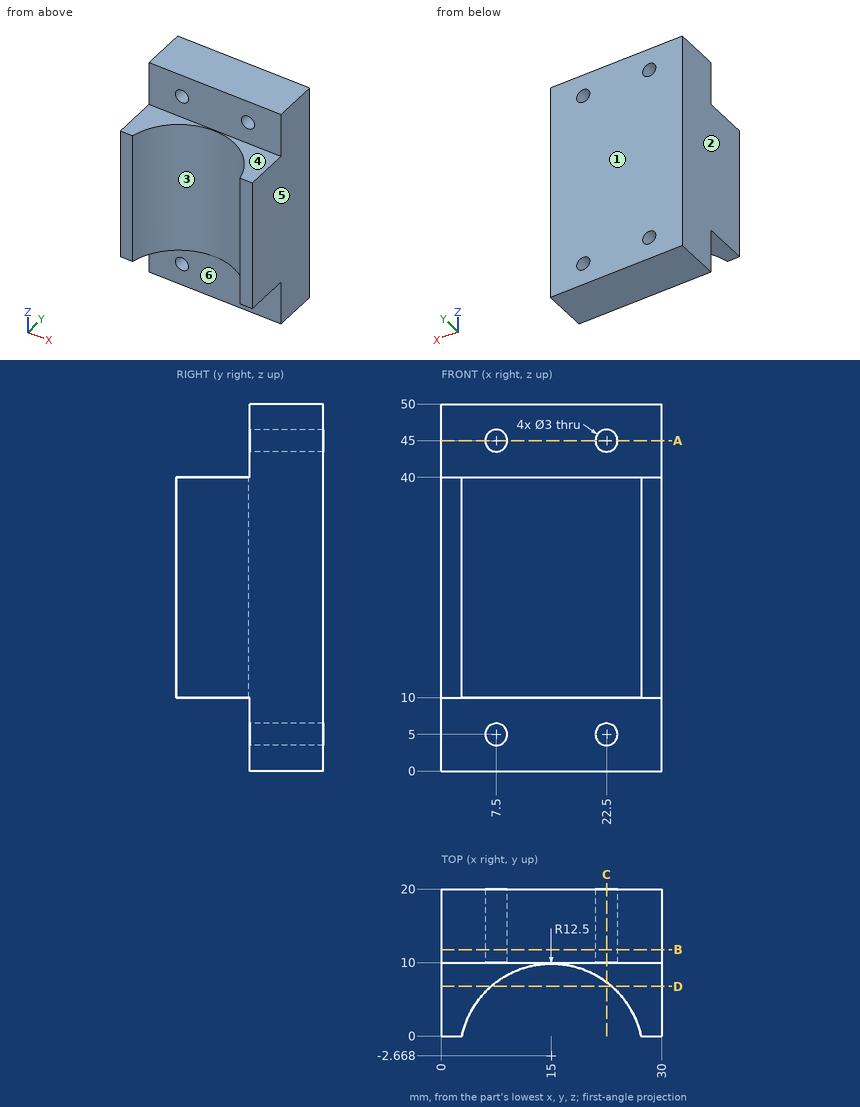
Input: dimensioned drawing with shaded views. Units: mm. Origin: part minimum x, y, z. A direction names the side the tool comes from. Give positions to 0.01 mm unless a question says otherwise; leave off trailing zeros. Write each loop counter-clockwise with the first axis right and the second up, starting at its lowest first coordinate (ties: lowest second). Pieces come first, ordered by that corner, then holes. Notation, with made-up numbers: M 14,72.5 L 35,72.5 A22 cw 35,102.5 Z; hole C 68,-40 d6. An arc over 180 degrees is marked long. Return JSON: item names as keys, results as strings. Group by question number.
1) Cut plane B-B, the plane y = 11.75. Output: boundary loops of the cut face in (x, z), plus the area to 3 significant figures.
2) Cut plane A-A, the plane z = 45. Output: boundary loops of the cut face in (x, y), plus the area to 3 significant figures.
3) Set-up query: the marked faces 4, 5 and 6. Return all of +Z, -Z, +X, -X, +Y, -Y with unobstructed straight access to the full face (end or side cutting, diameter ignored); none if empty.
4) Pin query (flat end, axial travel): P1, Ø5, axis at x = 8, y = 6, coming from the +Z side; P2, Ø6, axis at x = 3.5, y = 2.5, coming from the -Z side; P3, Ø12, axis at y = 15.5, z = 10.5, coming from the -X side; P4, Ø3, axis at x = 14.5, z = 6, coming from the -Y side. Return the tip coordinate at first contact, or that it passes through.
5) Pull-direction query (X, two-part tool) for the marked faces 1, 2 and 3; classes: pulls with the +X half, pulls with the -X half, needs draft (parallel to the pull), parting line crosses it, or undercut.
6) Material intervals for line 1 along Z through (x, y) = (22.5, 16.75); line 2 along Z through (x, y) = (6.75, 15); line 3 along Y through (x, z) = (10.5, 24), sorted ascending. Write a range as [from, to].
7) Cut plane D-D, the plane y = 6.75. Output: boundary loops of the cut face in (x, z).
8) Cut plane C-C, the plane x = 22.5. Output: boundary loops of the cut face in (y, z).
Recorded:
{
 "1": {"outline": "M 0,0 L 30,0 L 30,50 L 0,50 Z; hole C 7.5,5 d3; hole C 7.5,45 d3; hole C 22.5,5 d3; hole C 22.5,45 d3", "area": "1,470 mm²"},
 "2": {"outline": "M 0,10 L 6,10 L 6,20 L 0,20 Z; M 9,10 L 21,10 L 21,20 L 9,20 Z; M 24,10 L 30,10 L 30,20 L 24,20 Z", "area": "240 mm²"},
 "3": {"face 4": "+Z, +X, -X, -Y", "face 5": "+Z, -Z, +X, +Y, -Y", "face 6": "-Z, +X, -X, -Y"},
 "4": {"P1": "stops at z = 40", "P2": "stops at z = 10", "P3": "stops at x = 0", "P4": "stops at y = 10"},
 "5": {"face 1": "needs draft", "face 2": "pulls with the -X half", "face 3": "undercut"},
 "6": {"line 1": "z = [0, 3.5], [6.5, 43.5], [46.5, 50]", "line 2": "z = [0, 3.7], [6.3, 43.7], [46.3, 50]", "line 3": "y = [8.99, 20]"},
 "7": {"outline": "M 0,10 L 6.78,10 L 6.78,40 L 0,40 Z; M 23.22,10 L 30,10 L 30,40 L 23.22,40 Z"},
 "8": {"outline": "M 7.33,10 L 10,10 L 10,6.5 L 20,6.5 L 20,43.5 L 10,43.5 L 10,40 L 7.33,40 Z; M 10,0 L 20,0 L 20,3.5 L 10,3.5 Z; M 10,46.5 L 20,46.5 L 20,50 L 10,50 Z"}
}
